Model file for the job. Use its own axes, mm. A direction names the side the tool comes from. Give positions to 0.01 mm unless a question says otherwise; leave off trailing zeros. Loops run counter-clockwise (first coordinate to the right, second up) from the corner with the lowest first, then second, coordinate; pieces in that order, holes last. Notation, with made-up numbers: (-9.5, 51) - (30.5, 51) arc R17 cw to (30.5, 81) - close; hole circle Ø2 at (14.25, 3.25). An arc over 180 degrees is marked (long way). Use a Markdown table: item, result.
Autodesk Inventor part; units mm, degrees
ref_plane "Arbeitsebene2" through (3, 20, 8.35) normal (0, -1, 0) x (1, 0, 0)
ref_plane "Arbeitsebene3" through (0, 60, 8.35) normal (0, -1, 0) x (1, 0, 0)
ref_plane "Arbeitsebene4" through (3, 0, 11.35) normal (0, 0, -1) x (-1, 0, 0)
sketch "Skizze1" plane through (0, 0, 0) normal (0, 1, 0) x (-1, 0, 0)
  line L0 (0, 0) -> (-3, 0)
  line L1 (-3, 0) -> (-3, 23)
  line L2 (-3, 23) -> (-40, 23)
  line L3 (-40, 23) -> (-40, 26)
  line L4 (-40, 26) -> (0, 26)
  line L5 (0, 26) -> (0, 0)
  line L6 (0, -5.2) -> (0, 31.2)
  line L7 (8, 0) -> (-48, 0)
  point P0 (0, 0)
  dimension "d0" = 3
  dimension "d1" = 3
  dimension "d2" = 40
  dimension "d3" = 26
extrude "Extrusion1" add sketch "Skizze1" along normal blind 80
fillet "Rundung1" radius 6 1 edges at (0, 40, 26)
fillet "Rundung2" radius 4 1 edges at (3, 40, 23)
sketch "Skizze2" plane through (3, 0, 0) normal (1, 0, 0) x (0, 0, -1)
  arc A0 (-14.35, 24.35) -> (-14.35, 15.65) centre (-14.35, 20) ccw
  arc A1 (-8.35, 15.65) -> (-8.35, 24.35) centre (-8.35, 20) ccw
  line L0 (-14.35, 24.35) -> (-8.35, 24.35)
  line L1 (-8.35, 15.65) -> (-14.35, 15.65)
  line L2 (-31.2, 0) -> (5.2, 0)
  line L3 (0, 0) -> (0, 80)
  point P0 (-4, 20)
  dimension "d17" = 8.7
  dimension "d18" = 6
  dimension "d19" = 20
  dimension "d20" = 8.7
  dimension "d21" = 4
extrude "Extrusion2" cut sketch "Skizze2" against normal through all
ref_plane "Arbeitsebene1" through (0, 40, 0) normal (0, 1, 0) x (-1, 0, 0)
mirror "Spiegeln1" about plane through (0, 40, 0) normal (0, 1, 0) of "Extrusion2"
sketch "Skizze3" plane through (40, 0, 23) normal (0, 0, -1) x (-1, 0, 0)
  arc A0 (6.35, 24.35) -> (6.35, 15.65) centre (6.35, 20) ccw
  arc A1 (14.35, 15.65) -> (14.35, 24.35) centre (14.35, 20) ccw
  line L0 (6.35, 24.35) -> (14.35, 24.35)
  line L1 (14.35, 15.65) -> (6.35, 15.65)
  line L2 (48, 0) -> (-8, 0)
  line L3 (0, 0) -> (0, 80)
  point P0 (40, 0)
  point P1 (2, 20)
  dimension "d23" = 8.7
  dimension "d24" = 8
  dimension "d25" = 20
  dimension "d26" = 2
extrude "Extrusion3" cut sketch "Skizze3" against normal blind 10
mirror "Spiegeln2" about plane through (0, 40, 0) normal (0, 1, 0) of "Extrusion3"
ref_plane "Arbeitsebene2" through (3, 20, 8.35) normal (0, -1, 0) x (1, 0, 0)
ref_plane "Arbeitsebene3" through (0, 60, 8.35) normal (0, -1, 0) x (1, 0, 0)
ref_plane "Arbeitsebene4" through (3, 0, 11.35) normal (0, 0, -1) x (-1, 0, 0)
ref_plane "Arbeitsebene5" through (0, 20, 0) normal (0, -1, 0) x (1, 0, 0)
ref_plane "Arbeitsebene6" through (0, 60, 0) normal (0, 1, 0) x (1, 0, 0)
ref_plane "Arbeitsebene7" through (29.65, 0, 26) normal (1, 0, 0) x (0, 0, -1)
equation "\"Biegeradius\" = Stärke"
equation "\"BreiteBiegungsfreistellung\" = Stärke"
equation "\"TiefeBiegungsfreistellung\" = 0.5 * Stärke"
equation "\"GrößeEckenfreistellung\" = 4 * Stärke"
equation "\"MinimalRest\" = 2 * Stärke"
equation "\"Übergangsradius\" = Biegeradius"
equation "\"JacobiRadiusGröße\" = Biegeradius"
equation "\"Abstandsgröße\" = Stärke"
properties part number "Winkelblech"
(1) Slice it at B-B, the plane z = 13.5. Write the cut outline in (x, y).
Computed:
| item | result |
|---|---|
| outline | (0, 0) - (3, 0) - (3, 15.65) - (0, 15.65) - close; (0, 24.35) - (3, 24.35) - (3, 55.65) - (0, 55.65) - close; (0, 64.35) - (3, 64.35) - (3, 80) - (0, 80) - close |
(2) Drill centre lines: probe 1 along X at (y, z) = (50, 9); probe 2 along Z at (x, y) = (25, 4.5); probe 3 along Z at (x, y) = (2.5, 64). Where is each one in solid material? Low to high. Write a range as [from, to].
Computed:
| item | result |
|---|---|
| probe 1 | [0, 3] |
| probe 2 | [23, 26] |
| probe 3 | [0, 6.64], [16.06, 24.87] |
(3) Mould opens along X. For faces 5 (the flat face through (14, 0, 24)), 6 (the flat face through (40, 39, 24)), 7 (the flat face through (30, 64.35, 24)) say: pulls with the +X half, pulls with the -X half, needs draft (parallel to the pull), parting line crosses it, or undercut.
Computed:
| item | result |
|---|---|
| face 5 | needs draft |
| face 6 | pulls with the +X half |
| face 7 | undercut |
(4) Slice it at D-D, the plane z = 24.25. Write the cut outline in (x, y), plus the area to 3 significant figures.
Computed:
| item | result |
|---|---|
| outline | (1.76, 0) - (40, 0) - (40, 80) - (1.76, 80) - close; hole (25.65, 15.65) - (33.65, 15.65) arc R4.35 ccw to (33.65, 24.35) - (25.65, 24.35) arc R4.35 ccw to start; hole (25.65, 55.65) - (33.65, 55.65) arc R4.35 ccw to (33.65, 64.35) - (25.65, 64.35) arc R4.35 ccw to start |
| area | 2,800 mm² |
(5) Slice it at A-A, the plane y = 20. Write the cut outline in (x, z).
Computed:
| item | result |
|---|---|
| outline | (0, 0) - (3, 0) - (3, 4) - (0, 4) - close; (0, 18.7) - (3, 18.7) - (3, 19) arc R4 cw to (7, 23) - (21.3, 23) - (21.3, 26) - (6, 26) arc R6 ccw to (0, 20) - close; (38, 23) - (40, 23) - (40, 26) - (38, 26) - close |
(6) Slice it at C-C, the plane y = 33. Write the cut outline in (x, z).
Computed:
| item | result |
|---|---|
| outline | (0, 0) - (3, 0) - (3, 19) arc R4 cw to (7, 23) - (40, 23) - (40, 26) - (6, 26) arc R6 ccw to (0, 20) - close |
(7) Pin check, flat tip, straight feed: P1, Ø10, axis at x = 28, y = 47.5, coming from the -Z side. Stop position of the tip, or through.
Computed:
| item | result |
|---|---|
| P1 | z = 23 |
(8) 3-axis set-ups, long thin cutter, end or side, ignore diameter. For faces 1 (the flat face through (23, 39, 26)), 2 (the cylindrical face through (1.5, 20.1, 18.7)), 3 (the flat face through (23, 39, 23)), 4 (the flat face through (30, 15.65, 24)): which of +Z, -Z, +X, -X, +Y, -Y reach the whole face in a straight line?
Computed:
| item | result |
|---|---|
| face 1 | +Z, +X, -X, +Y, -Y |
| face 2 | +X, -X |
| face 3 | -Z, +X, +Y, -Y |
| face 4 | +Z, -Z |
